Design review of the part built by this model. Coordinates are the model's own, in mm. A direction names the side the tool comes from. Give positions to 0.01 mm unless a question says otherwise; leave off trailing zeros. Loops run counter-clockwise (first coordinate to the right, second up) from the corner with the lowest first, then second, coordinate; pieces in that order, holes last. Notation, with made-up numbers: (51.5, -2.75) - (96.5, -2.75) arc R24 cw to (96.5, 7.25) - close; hole circle Ø1 at (65.25, -2.75). An arc over 180 degrees is marked (long way). Put each result on its own line as item: value. Start each with the question number.
```python
from build123d import *

# Parameters (mm, degrees)
SKETCH1_W                      = 125
SKETCH1_H                      = 70
BOSS_EXTRUDE1_DEPTH            = 3.175
F_10_0_10_DIAMETER_HOLE1_D     = 10
F_10_0_10_DIAMETER_HOLE1_DEPTH = 3.175
F_8_0_8_DIAMETER_HOLE1_D       = 8
F_8_0_8_DIAMETER_HOLE1_DEPTH   = 3.175
CUT_EXTRUDE1_DEPTH             = 4.175


with BuildPart() as part:
    # Sketch1 → Boss-Extrude1 (new body)
    with BuildSketch(Plane(origin=(0, 0, 0), x_dir=(1, 0, 0), z_dir=(0, 1, 0))):
        Rectangle(SKETCH1_W, SKETCH1_H)
    extrude(amount=BOSS_EXTRUDE1_DEPTH)

    # Ø10.0 (10) Diameter Hole1
    with Locations(Plane(origin=(0, 3.175, 0), x_dir=(1, 0, 0), z_dir=(0, 1, 0))):
        with Locations((-12.5, 0), (5.544081657, -20.339852315)):
            Hole(F_10_0_10_DIAMETER_HOLE1_D / 2, depth=F_10_0_10_DIAMETER_HOLE1_DEPTH)

    # Ø8.0 (8) Diameter Hole1
    with Locations(Plane(origin=(0, 3.175, 0), x_dir=(1, 0, 0), z_dir=(0, 1, 0))):
        with Locations((2.300160709, 19.912165142), (-12.5, 0)):
            Hole(F_8_0_8_DIAMETER_HOLE1_D / 2, depth=F_8_0_8_DIAMETER_HOLE1_DEPTH)

    # Sketch7 → Cut-Extrude1 (cut, through all)
    with BuildSketch(Plane(origin=(0, 3.175, 0), x_dir=(1, 0, 0), z_dir=(0, 1, 0))):
        Polygon((-62.5, 35), (-59.325, 35), (-59.325, 10), (-59.325, -10), (-62.5, -10), (-62.5, 10), align=None)
        Polygon((62.5, 35), (59.325, 35), (59.325, 10), (59.325, -10), (62.5, -10), (62.5, 10), align=None)
    extrude(amount=-CUT_EXTRUDE1_DEPTH, mode=Mode.SUBTRACT)


solid = part.part
```
Item 1: For P1, Ø6, axis at x = 5.54, z = 20.34, coming from the -Y side; P2, Ø1, axis at x = -61.5, y = 1, coming from the -Z side, all flat-tipped, find the tip position at first contact; note any pin that passes through.
Item 2: Mouldability with a two-part tool opening along Z and no side actions: class faces 4 (the cylindrical face through (2.82, 1.57, -23.88)), 5 (the flat face through (-59.325, 2, -12)), 6 (the flat face through (-1, 2, 35)) as pulls with the +Z half, pulls with the -Z half, needs draft (parallel to the pull), parting line crosses it, or undercut.
Item 3: Consider section B-B (z = 0). State the section outline as (x, y) points (3 decimals).
Item 4: For L1, parallel to Z at x = 2, y = 1.3; L2, parallel to Z at x = -12.5, y = 1.95; L3, parallel to X at y = 1.3, z = 20.5, list the stretches that pass through material, from the lowest coordinate up. Write a range as from..to.
Item 5: Machinability: for faces 1 (the cylindrical face through (9.5, 1.6, 23.4)), 2 (the flat face through (-61, 2, 10)), 3 (the flat face through (59.325, 2, -13)), which of the approach directions +Z, -Z, +X, -X, +Y, -Y give a long, thin tool a straight path to every point of the face, cutting with its end or side? Answer none if there is none.
Item 6: Consider section A-A (x = -12.5). State the section outline as (y, z) points (3 decimals).
Item 7: Consider section C-C (y = 1.75). State the section outline as (x, z) points (3 decimals).
Geometry says:
1. P1: passes through
1. P2: stops at z = 10
2. face 4: undercut
2. face 5: needs draft
2. face 6: pulls with the +Z half
3. outline: (-59.325, 0) - (-17.5, 0) - (-17.5, 3.175) - (-59.325, 3.175) - close; (-7.5, 0) - (59.325, 0) - (59.325, 3.175) - (-7.5, 3.175) - close
4. L1: z = -35..-23.9, -15.92..16.81, 23.87..35
4. L2: z = -35..-5, 5..35
4. L3: x = -62.5..0.55, 10.54..62.5
5. face 1: +Y, -Y
5. face 2: -Z, -X, +Y, -Y
5. face 3: -Z, +X, +Y, -Y
6. outline: (0, -35) - (3.175, -35) - (3.175, -5) - (0, -5) - close; (0, 5) - (3.175, 5) - (3.175, 35) - (0, 35) - close
7. outline: (-62.5, 10) - (-59.325, 10) - (-59.325, -35) - (59.325, -35) - (59.325, 10) - (62.5, 10) - (62.5, 35) - (-62.5, 35) - close; hole circle Ø10 at (-12.5, 0); hole circle Ø8 at (2.3, -19.912); hole circle Ø10 at (5.544, 20.34)
